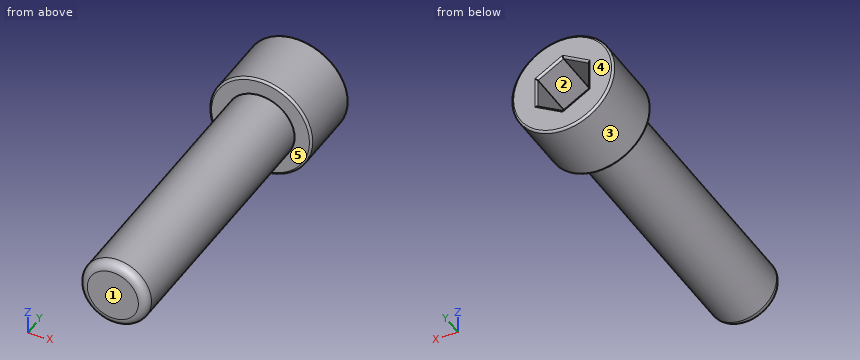
from build123d import *

# Parameters (mm, degrees)
F0_R     = 4
F1_DEPTH = 32
F0_R_2   = 6
F2_DEPTH = 8
F4_DEPTH = 6
F5_R     = 0.25
F6_R     = 1


with BuildPart() as f1:
    # F0 (on Front) → F1 (new body)
    with BuildSketch(Plane.XZ):
        Circle(F0_R)
    extrude(amount=F1_DEPTH)

    # F0 (on Front) → F2 (join)
    with BuildSketch(Plane.XZ):
        Circle(F0_R_2)
        Circle(F0_R, mode=Mode.SUBTRACT)
        Circle(F0_R)
    extrude(amount=-F2_DEPTH)

    # F3 (on face) → F4 (cut)
    with BuildSketch(Plane(origin=(0, 8, 0), x_dir=(-1, 0, 0), z_dir=(0, 1, 0))):
        Polygon((-3, 1.732051), (-3, -1.732051), (0, -3.464102), (3, -1.732051), (3, 1.732051), (0, 3.464102), align=None)
    extrude(amount=-F4_DEPTH, mode=Mode.SUBTRACT)

    # F5
    f5_edges = [f1.edges().sort_by_distance(p)[0] for p in [
        (1.5, 8, -2.598076),
        (-1.5, 8, -2.598076),
        (-3, 8, 0),
        (-1.5, 8, 2.598076),
        (1.5, 8, 2.598076),
        (3, 8, 0),
        (-6, 8, 0),
        (1.5, 2, -2.598076),
        (-1.5, 2, -2.598076),
        (3, 2, 0),
        (1.5, 2, 2.598076),
        (-1.5, 2, 2.598076),
        (-3, 2, 0),
        (-6, 0, 0),
    ]]
    fillet(f5_edges, radius=F5_R)

    # F6
    f6_edges = [f1.edges().sort_by_distance(p)[0] for p in [
        (-4, -32, 0),
    ]]
    fillet(f6_edges, radius=F6_R)


solid = f1.part
Geometry check sheet. Reference: the model listing, model coordinates, mm. Face numbers are marked on the shaded views. A direction names the side the tool comes from. Round coordinates to 2 decimals unless told otherwise and drop trailing zeros. Loops run counter-clockwise (first coordinate to the right, second up) from the corner with the lowest first, then second, coordinate; pieces in that order, holes last. Notation, with made-up numbers: (81, 40.5) - (127, 40.5) arc R23 cw to (127, 61.5) - close; hole circle Ø5 at (-37.5, -31.5). An arc over 180 degrees is marked (long way). One line per question, with ' | ' between items. Start each with the question number.
1. Depth check by flat-ended pin: pin 1 (3 mm diameter, centred on y = -15.5, z = -0.5, fed in from -X); pin 2 (3 mm diameter, centred on x = 3, y = 1, fed in from +Z). Enter the tip coordinate at first touch or a pass-through.
2. Tool access check on the marked faces 4 and 5. Record the directions out of +Z, -Z, +X, -X, +Y, -Y that give a thin tool (end or side, any length) a straight path to the whole face; none if there is none.
3. Scan lines: line 1 (Y direction, x = 2.25, z = -1); line 2 (Y direction, x = 0.75, z = 4.75); line 3 (X direction, y = 2.5, z = -0.5). Record each from-to range of solid material in increasing order. Write a range as [from, to].
4. Cross-section at A-A on z = 0. Record the cut outline in (x, y).
5. Cross-section at B-B on y = -25.5. Record the cut outline in (x, z), then the cut area to 3 significant figures.
6. Draft check along Z on the marked faces 1, 2 and 3. Enter one of: released by +Z, released by -Z, zero draft, split by the parting line, or undercut.
Taken from the geometry:
1) pin 1: x = -4 | pin 2: z = 5.81
2) face 4: +Z, -Z, +X, -X, +Y | face 5: -Y
3) line 1: [-32, 2] | line 2: [0, 8] | line 3: [-5.98, -3], [3, 5.98]
4) outline: (-6, 0.25) arc R0.25 ccw to (-5.75, 0) - (-4, 0) - (-4, -31) arc R1 ccw to (-3, -32) - (3, -32) arc R1 ccw to (4, -31) - (4, 0) - (5.75, 0) arc R0.25 ccw to (6, 0.25) - (6, 7.75) arc R0.25 ccw to (5.75, 8) - (3.25, 8) arc R0.25 ccw to (3, 7.75) - (3, 2.25) arc R0.25 cw to (2.75, 2) - (-2.75, 2) arc R0.25 cw to (-3, 2.25) - (-3, 7.75) arc R0.25 ccw to (-3.25, 8) - (-5.75, 8) arc R0.25 ccw to (-6, 7.75) - close
5) outline: circle Ø8 at (0, 0) | area: 50.3 mm²
6) face 1: zero draft | face 2: undercut | face 3: split by the parting line
